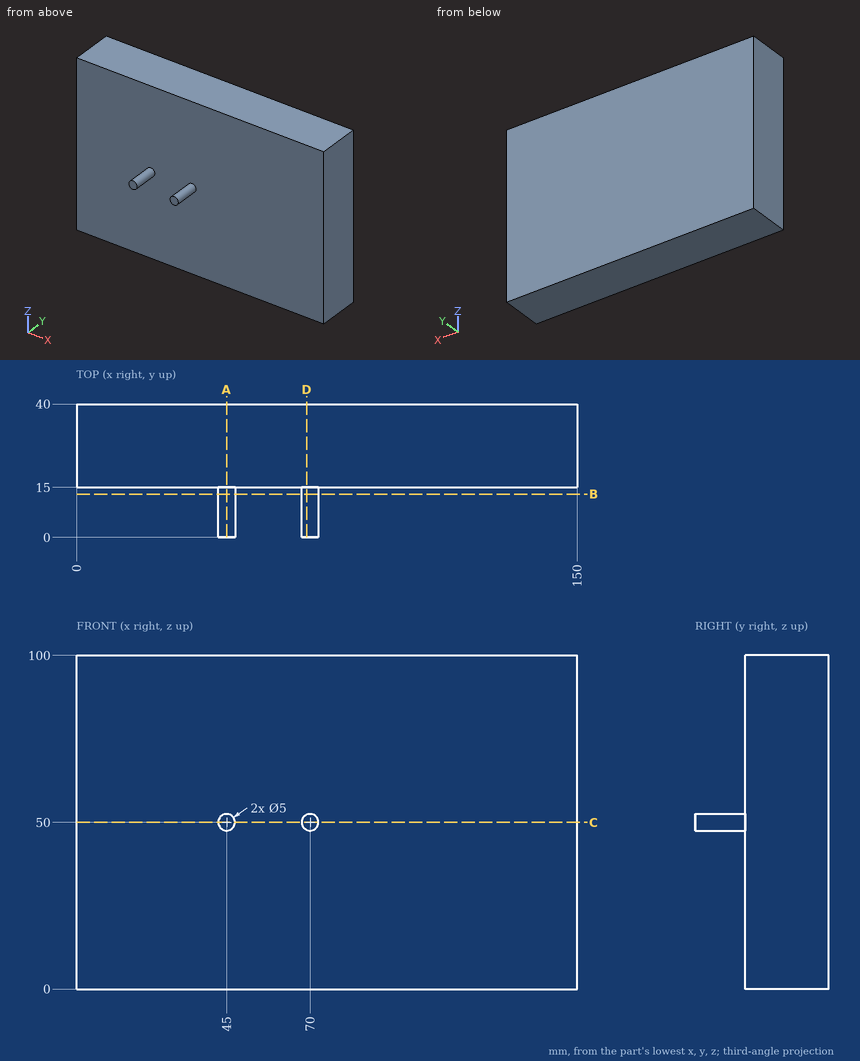
Input: dimensioned drawing with shaded views. Units: mm. Origin: part minimum x, y, z. Give positions to 0.01 mm unless a question says otherwise; leave off trailing zeros. Write each loop counter-clockwise with the first axis right and the second up, starting at its lowest first coordinate (ties: lowest second). Pieces come first, ordered by that corner, then holes.
Q1. First-contact query: P1, Ø5, axis at x = 32, z = 46.5, coming from the -Y side; P2, Ø1.5, axis at x = 31.5, y = 14, coming from the -Z side. Flat tips, straight axial feed; report the tip coordinate or a pass-through.
Q2. Section B-B, the plane y = 13. Output: boundary loops of the cut face in (x, z), plus the area to 3 significant figures.
Q3. Section D-D, the plane x = 69. Output: boundary loops of the cut face in (y, z), plus the area to 3 significant figures.
Q4. Material intervals for probe 1 along Y at (x, z) = (14, 24.5), sorted ascending.
Q5. Section C-C, the plane z = 50. Output: boundary loops of the cut face in (x, y), plus the area to 3 significant figures.
Q6. Section A-A, the plane x = 45. Output: boundary loops of the cut face in (y, z).
Filled in:
1. P1: stops at y = 15
1. P2: passes through
2. outline: circle Ø5 at (45, 50); circle Ø5 at (70, 50)
2. area: 39.3 mm2
3. outline: (0, 47.71) - (15, 47.71) - (15, 0) - (40, 0) - (40, 100) - (15, 100) - (15, 52.29) - (0, 52.29) - close
3. area: 2,570 mm2
4. probe 1: y = 15 to 40
5. outline: (0, 15) - (42.5, 15) - (42.5, 0) - (47.5, 0) - (47.5, 15) - (67.5, 15) - (67.5, 0) - (72.5, 0) - (72.5, 15) - (150, 15) - (150, 40) - (0, 40) - close
5. area: 3,900 mm2
6. outline: (0, 47.5) - (15, 47.5) - (15, 0) - (40, 0) - (40, 100) - (15, 100) - (15, 52.5) - (0, 52.5) - close
